Answer from the drawing. Dimensions are ordinates in mm from the lowest x, y and z of the part. Give positions to 0.01 mm unless a question says otherwise; leave off trailing zeros. Order: outer loops, then holes, each group sorted by start corner. A loop starts at its lowest first (then second) coordinate and runs counter-clockwise, first axis right, second up. Notation, with made-up numbers: M 44.25,57 L 89.25,57 A11 ccw 89.25,66 Z; hole C -4,73.5 d4. An arc over 180 degrees is marked long. One line per item, written item: value.
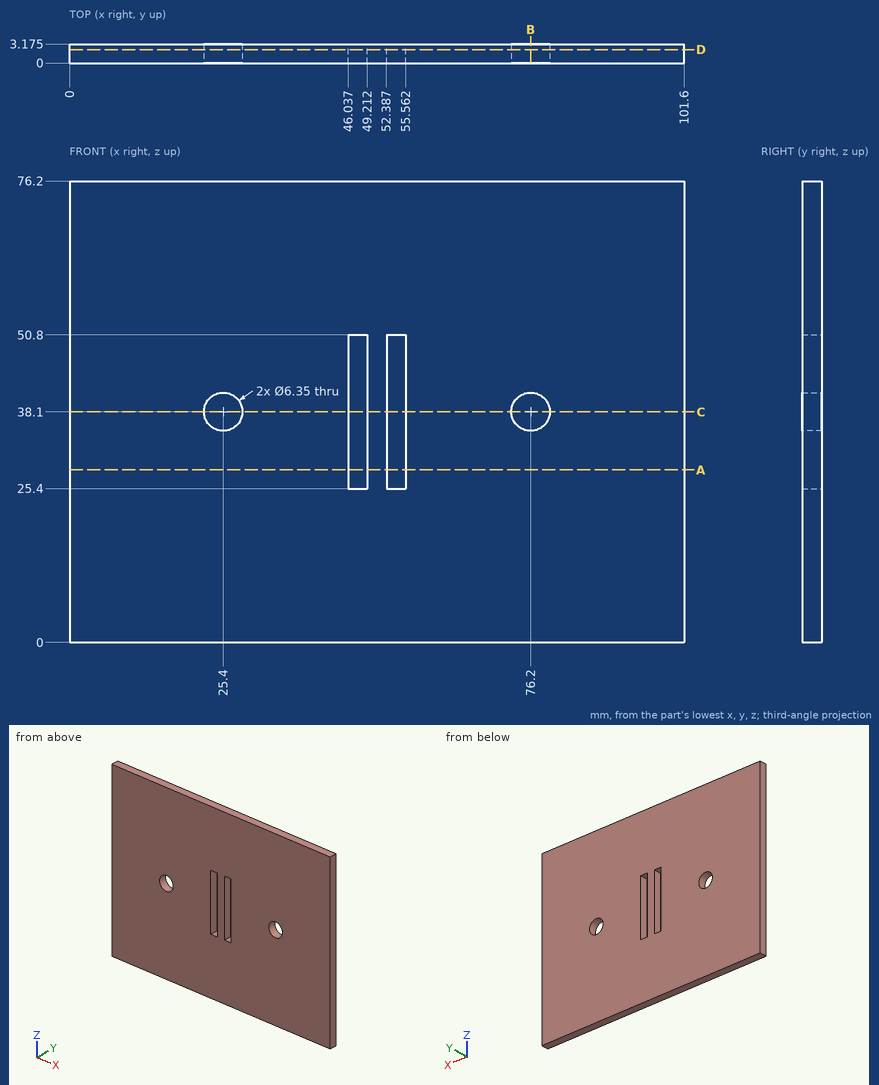
(1) Section C-C, the plane z = 38.1 is taken. Give the vertices of the cut face in (x, y) (1 decimal).
Findings:
outline: M 0,0 L 22.2,0 L 22.2,3.2 L 0,3.2 Z; M 28.6,0 L 46,0 L 46,3.2 L 28.6,3.2 Z; M 49.2,0 L 52.4,0 L 52.4,3.2 L 49.2,3.2 Z; M 55.6,0 L 73,0 L 73,3.2 L 55.6,3.2 Z; M 79.4,0 L 101.6,0 L 101.6,3.2 L 79.4,3.2 Z
(2) Section B-B, the plane x = 76.2 is taken. Give the vertices of the cut face in (y, z) (1 decimal).
Findings:
outline: M 0,0 L 3.2,0 L 3.2,34.9 L 0,34.9 Z; M 0,41.3 L 3.2,41.3 L 3.2,76.2 L 0,76.2 Z
(3) Section D-D, the plane y = 2.25 is taken. Give the number of separate pieces and of enclosed holes in the cut face, then the cut area to 3 significant figures.
Findings:
separate pieces: 1
enclosed holes: 4
area: 7,520 mm^2
(4) Section A-A, the plane z = 28.5 is taken. Give the vertices of the cut face in (x, y) (1 decimal).
Findings:
outline: M 0,0 L 46,0 L 46,3.2 L 0,3.2 Z; M 49.2,0 L 52.4,0 L 52.4,3.2 L 49.2,3.2 Z; M 55.6,0 L 101.6,0 L 101.6,3.2 L 55.6,3.2 Z
(5) Find the intervals of material crossed by probe 1 along X at (y, z) = (1.4, 49.5); probe 2 along X at (y, z) = (1.65, 38.1) (1 decimal), in increasing order. Write a range as from..to.
Findings:
probe 1: x = 0..46.04, 49.21..52.39, 55.56..101.6
probe 2: x = 0..22.2, 28.6..46, 49.2..52.4, 55.6..73, 79.4..101.6
